Verification items for the finished model (mm, model axes). Face numbers are marked on the shaded views. A direction names the side the tool comes from. Round coordinates to 2 decimals unless told otherwise and drop trailing zeros. Write each loop counter-clockwise with the first axis right and the second up, starting at its lowest first coordinate (ties: lowest second). Pieces come first, ordered by that corner, then holes. Notation, with made-up numbers: (49, 7.25) -> (88, 7.25) arc R9 ccw to (88, 13.25) -> close; hole circle Ø5 at (-40, -31). An arc over 180 degrees is marked (long way). Answer as a JSON object with one key per item and string values. Group by question number.
(1) Sectioned sample at D-D on x = 0. Count the separate pieces of the cut face and the enclosed holes in it, and give its area (3 significant figures).
(2) Draft check along X on the marked faces 1, 2 and 3. Enter one of: released by +X, released by -X, zero draft, split by the parting line, or undercut.
(3) Sectioned sample at C-C on y = 8.5. Record the cut outline in (x, z).
(4) Gauge pin test, flat ends, axial feed: pin 1 Ø4 at (x, z) = (-14, -1.5) entering from -Y; pin 2 Ø1 at (x, y) = (11, -15) entering from -Z; pin 3 Ø0.6 at (x, z) = (-3, -1.5) entering from -Y; pin 4 Ø8 at (x, z) = (-12, -7.5) entering from -Y. Record the tip position at first contact, or that the pin passes through.
(5) Sectioned sample at A-A on x = 14. Record the cut outline in (y, z).
(6) Scan lines: L1, parallel to X at y = -25.95, z = 5.5; L2, parallel to Y at x = -14, z = -0.85; L3, parallel to Y at x = -18.5, z = 5.5. Record each from-to range of solid material in increasing order. Write a range as from..to.
(7) Set-up check for the marked faces 4, 5 and 6: record each of +Z, -Z, +X, -X, +Y, -Y from which the full face is reachable in a straight line by a thin tool's end or side.
(8) Sectioned sample at B-B on x = 10. Record the cut outline in (y, z).
```python
from build123d import *

# Parameters (mm, degrees)
SKETCH_1_W             = 36
SKETCH_1_H             = 36
EXTRUDE_1_DEPTH        = 11
SKETCH_2_W             = 32
SKETCH_2_H             = 32
SKETCH_2_R             = 1.25
EXTRUDE_2_DEPTH        = 2
EXTRUDE_START          = -11
SKETCH_3_R             = 7
EXTRUDE_3_DEPTH        = 22.2
SKETCH_4_W             = 1
SKETCH_4_H             = 2
SKETCH_5_R             = 5
CUT_EXTRUDE_1_DEPTH    = 0.9
EXTRUDE_START_2        = 19.25
SKETCH_6_R             = 0.75
EXTRUDE_4_DEPTH        = 1.25
EXTRUDE_5_DEPTH        = 37.25
SKETCH_9_R             = 12.5
SKETCH_9_R_2           = 1
EXTRUDE_6_DEPTH        = 1
CUT_EXTRUDE_2_DEPTH    = 2
SKETCH_10_R            = 0.75
EXTRUDE_7_DEPTH        = 1.25
HOLE_WIZARD_M2_1_D     = 1.6
HOLE_WIZARD_M2_1_DEPTH = 2
HOLE_WIZARD_M2_1_TIP   = 0.480688495


with BuildPart() as part:
    # 草图1 → 凸台-拉伸1 (new body)
    with BuildSketch(Plane.XY):
        Rectangle(SKETCH_1_W, SKETCH_1_H)
    extrude(amount=EXTRUDE_1_DEPTH)

    # 草图2 → 凸台-拉伸2 (add)
    with BuildSketch(Plane(origin=(0, 0, 0), x_dir=(-1, 0, 0), z_dir=(0, 0, -1))):
        Rectangle(SKETCH_2_W, SKETCH_2_H)
        with Locations((-14, 14)):
            Circle(SKETCH_2_R, mode=Mode.SUBTRACT)
        with Locations(Location((14, -14, 0), (0, 0, 180))):
            Circle(SKETCH_2_R, mode=Mode.SUBTRACT)
        with Locations(Location((14, 14, 0), (0, 0, 180))):
            Circle(SKETCH_2_R, mode=Mode.SUBTRACT)
        with Locations((-14, -14)):
            Circle(SKETCH_2_R, mode=Mode.SUBTRACT)
    extrude(amount=EXTRUDE_2_DEPTH)

    # 草图3 → 凸台-拉伸3 (add)
    with BuildSketch(Plane(origin=(0, 0, 0), x_dir=(-1, 0, 0), z_dir=(0, 0, -1)).offset(EXTRUDE_START)):
        with Locations(Location((0, 0, 0), (0, 0, 180))):
            Circle(SKETCH_3_R)
    extrude(amount=EXTRUDE_3_DEPTH)

    # 草图4 → 切除-旋转1 (revolve, cut)
    with BuildSketch(Plane(origin=(0, 0, 0), x_dir=(0, 0, -1), z_dir=(1, 0, 0)), mode=Mode.PRIVATE) as cut_revolve_1_sk:
        with Locations((9, 7)):
            Rectangle(SKETCH_4_W, SKETCH_4_H)
    revolve(cut_revolve_1_sk.sketch.rotate(Axis((0, 0, 0), (0, 0, -1)), 90), axis=Axis((0, 0, 0), (0, 0, -1)), mode=Mode.SUBTRACT)

    # 草图5 → 切除-拉伸1 (cut)
    with BuildSketch(Plane(origin=(0, 0, -11.2), x_dir=(-1, 0, 0), z_dir=(0, 0, -1))):
        Circle(SKETCH_5_R)
    extrude(amount=-CUT_EXTRUDE_1_DEPTH, mode=Mode.SUBTRACT)

    # 草图6 → 凸台-拉伸4 (add)
    with BuildSketch(Plane(origin=(0, 0, 0), x_dir=(0, 0, -1), z_dir=(1, 0, 0)).offset(EXTRUDE_START_2)):
        with BuildLine():
            Line((-0.75, -26.5), (-3.008892206, 0.210670265))
            ThreePointArc((-3.008892206, 0.210670265), (-5.5, 2.5), (-7.991107794, 0.210670265))
            Line((-7.991107794, 0.210670265), (-10.25, -26.5))
            Line((-10.25, -26.5), (-0.75, -26.5))
        make_face()
        with Locations((-5.5, 0)):
            Circle(SKETCH_6_R, mode=Mode.SUBTRACT)
    extrude(amount=-EXTRUDE_4_DEPTH)

    # 草图7 → 凸台-拉伸5 (add)
    with BuildSketch(Plane.ZY.offset(-18)):
        Polygon((0.834568908, -25.5), (10.165431092, -25.5), (10.25, -26.5), (0.75, -26.5), align=None)
    extrude(amount=EXTRUDE_5_DEPTH)

    # 草图9 → 凸台-拉伸6 (add)
    with BuildSketch(Plane.XZ.offset(26.5)):
        with Locations((0, 5.5)):
            Circle(SKETCH_9_R)
        with Locations((0, 5.5)):
            Circle(SKETCH_9_R_2, mode=Mode.SUBTRACT)
        with BuildLine():
            ThreePointArc((4.850909325, 14.244637141), (0, 15.5), (-4.850909325, 14.244637141))
            ThreePointArc((-4.850909325, 14.244637141), (-4.258969051, 12.844732491), (-3.274022071, 11.687146312))
            ThreePointArc((-3.274022071, 11.687146312), (0, 12.5), (3.274022071, 11.687146312))
            ThreePointArc((3.274022071, 11.687146312), (4.258969051, 12.844732491), (4.850909325, 14.244637141))
        make_face(mode=Mode.SUBTRACT)
        with BuildLine():
            ThreePointArc((-4.850909325, -3.244637141), (-4.258969051, -1.844732491), (-3.274022071, -0.687146312))
            ThreePointArc((-3.274022071, -0.687146312), (0, -1.5), (3.274022071, -0.687146312))
            ThreePointArc((3.274022071, -0.687146312), (4.258969051, -1.844732491), (4.850909325, -3.244637141))
            ThreePointArc((4.850909325, -3.244637141), (0, -4.5), (-4.850909325, -3.244637141))
        make_face(mode=Mode.SUBTRACT)
    extrude(amount=-EXTRUDE_6_DEPTH)

    # 草图8 → 切除-拉伸2 (cut)
    with BuildSketch(Plane.XZ.offset(26.5)):
        with BuildLine():
            Line((6.25, 7), (11.25, 7))
            ThreePointArc((11.25, 7), (12.75, 5.5), (11.25, 4))
            Line((11.25, 4), (6.25, 4))
            ThreePointArc((6.25, 4), (4.75, 5.5), (6.25, 7))
        make_face()
    cut_extrude_2 = extrude(amount=-CUT_EXTRUDE_2_DEPTH, mode=Mode.SUBTRACT)

    # 草图10 → 凸台-拉伸7 (add)
    with BuildSketch(Plane.ZY.offset(18)):
        with BuildLine():
            Line((3.008892206, 0.210670265), (0.75, -26.5))
            Line((0.75, -26.5), (10.25, -26.5))
            Line((10.25, -26.5), (7.991107794, 0.210670265))
            ThreePointArc((7.991107794, 0.210670265), (5.5, 2.5), (3.008892206, 0.210670265))
        make_face()
        with Locations(Location((5.5, 0, 0), (0, 0, 180))):
            Circle(SKETCH_10_R, mode=Mode.SUBTRACT)
    extrude(amount=EXTRUDE_7_DEPTH)

    # 镜向3: 切除-拉伸2 across plane
    add(cut_extrude_2.mirror(Plane(origin=(0, 0, 0), x_dir=(0, 0, 1), z_dir=(1, 0, 0))), mode=Mode.SUBTRACT)

    # M2 螺纹孔的螺纹孔钻头1
    with Locations(Plane(origin=(0, -26.5, 0), x_dir=(-1, 0, 0), z_dir=(0, -1, 0))):
        with Locations((0, -5.5)):
            Hole(HOLE_WIZARD_M2_1_D / 2, depth=HOLE_WIZARD_M2_1_DEPTH)
            with Locations((0, 0, -(HOLE_WIZARD_M2_1_DEPTH + HOLE_WIZARD_M2_1_TIP / 2))):  # 118° drill point
                Cone(0, HOLE_WIZARD_M2_1_D / 2, HOLE_WIZARD_M2_1_TIP, mode=Mode.SUBTRACT)


solid = part.part
```
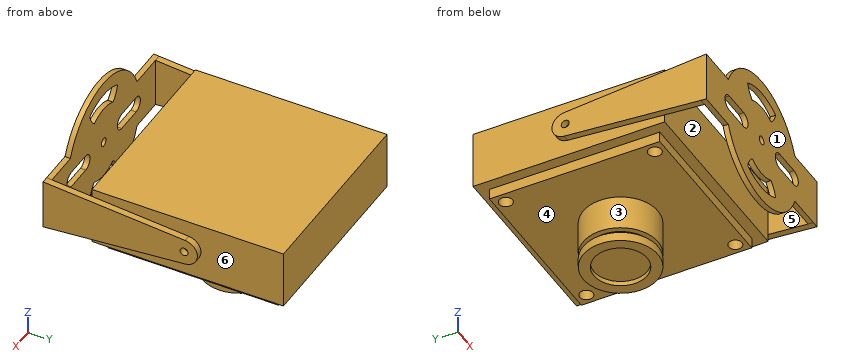
Computed values:
{
 "1": {"separate pieces": "5", "enclosed holes": "0", "area": "595 mm2"},
 "2": {"face 1": "zero draft", "face 2": "undercut", "face 3": "split by the parting line"},
 "3": {"outline": "(-18, 0) -> (-16, 0) -> (-16, -2) -> (16, -2) -> (16, 0) -> (18, 0) -> (18, 11) -> (-18, 11) -> close"},
 "4": {"pin 1": "y = -18", "pin 2": "z = -2", "pin 3": "y = -16", "pin 4": "through"},
 "5": {"outline": "(-26.5, 0.75) -> (-25.5, 0.83) -> (-25.5, 10.17) -> (-26.5, 10.25) -> close; (-18, 0) -> (-16, 0) -> (-16, -2) -> (-15.25, -2) -> (-15.25, 0) -> (-12.75, 0) -> (-12.75, -2) -> (12.75, -2) -> (12.75, 0) -> (15.25, 0) -> (15.25, -2) -> (16, -2) -> (16, 0) -> (18, 0) -> (18, 11) -> (-18, 11) -> close"},
 "6": {"L1": "-19.25..-12.75, -4.75..-0.8, 0.8..4.75, 12.75..19.25", "L2": "-16..-15.25, -12.75..12.75, 15.25..16", "L3": "-26.5..-0.75, 0.75..2.5"},
 "7": {"face 4": "-Z", "face 5": "+Z, -Z", "face 6": "+X, +Y"},
 "8": {"outline": "(-26.5, -2) -> (-25.5, -2) -> (-25.5, 4) -> (-26.5, 4) -> close; (-26.5, 7) -> (-25.5, 7) -> (-25.5, 13) -> (-26.5, 13) -> close; (-18, 0) -> (-16, 0) -> (-16, -2) -> (16, -2) -> (16, 0) -> (18, 0) -> (18, 11) -> (-18, 11) -> close"}
}
